from build123d import *

# Parameters (mm, degrees)
F0_R     = 1.875
F1_DEPTH = 11
F2_W     = 17.4188611699
F2_H     = 4.25
F3_DEPTH = 5


# Not quite as in the source:
# - a feature names something its author has since deleted; it is built from what else it names


with BuildPart() as f1:
    # F0 (on Top) → F1 (new body)
    with BuildSketch(Plane.XY):
        with BuildLine():
            ThreePointArc((1.5092688833, -2.1477272727), (2.3294265194, -1.2101227585), (2.625, 0))
            ThreePointArc((2.625, 0), (2.347022952, 1.1756310061), (1.5719651333, 2.1022727273))
            ThreePointArc((1.5719651333, 2.1022727273), (-2.6247144161, 0.0387199415), (1.5092688833, -2.1477272727))
        make_face()
        Circle(F0_R, mode=Mode.SUBTRACT)
        with BuildLine():
            ThreePointArc((1.5719651333, 2.1022727273), (2.347022952, 1.1756310061), (2.625, 0))
            ThreePointArc((2.625, 0), (2.3294265194, -1.2101227585), (1.5092688833, -2.1477272727))
            Line((1.5092688833, -2.1477272727), (24.9281300532, -2.1477272727))
            Line((24.9281300532, -2.1477272727), (24.9281300532, 2.1022727273))
            Line((24.9281300532, 2.1022727273), (1.5719651333, 2.1022727273))
        make_face()
    extrude(amount=F1_DEPTH)

    # F2 (on face) → F3 (join)
    with BuildSketch(Plane.XY.offset(11)):
        with Locations((16.2186994682, -0.0227272727)):
            Rectangle(F2_W, F2_H)
    extrude(amount=F3_DEPTH)


solid = f1.part
Can you work these out from the model? Positions are in its coordinate system, mm. A direction names the side the tool comes from. Give positions to 0.01 mm unless a question says otherwise; leave off trailing zeros. Loops run counter-clockwise (first coordinate to the right, second up) from the corner with the lowest first, then second, coordinate; pieces in that order, holes last. Notation, with made-up numbers: M 28.5,29.5 L 57.5,29.5 A21 ccw 57.5,63.5 Z; hole C 24,18.25 d3. An arc over 180 degrees is marked long. One line per item, written item: value. Start each with the question number.
1) If we section it at A-A, the plane y = 0: Write out the boundary of the cut face in (x, z) (3 decimals).
2) I'm going to push flat-ended pins straight in: pin 1 (1 mm diameter, centred on x = 10.5, y = 0, fed in from -Z); pin 2 (5 mm diameter, centred on x = 9.5, z = 10, fed in from -Y); pin 3 (1.5 mm diameter, centred on y = -2, z = 5.5, fed in from -X). Where does each tip first touch, or does it pass through?
3) If we section it at D-D, the plane x = 8.5: Write out the boundary of the cut face in (y, z).
4) If I drill on line 1 (Y direction, x = 14.5, z = 6); line 2 (Z direction, x = 6.25, y = 1.6); line 3 (X direction, y = -0.7, z = 15), over which ranges is the centre line in solid material (lowest first)? Write a range as [from, to].
5) If we section it at C-C, the plane z = 2.25: Write out the boundary of the cut face in (x, y) (3 decimals).
6) Thinking about a two-plate mould opening in X: for faces 4 (the face through (16, 0, 16)), 5 (the face through (-1.873, 0.082, 5.423)), 6 (the face through (-2.622, 0.119, 5.423)), which applies, +X half, -X half, draft (parallel to the pull), parting line (faces both ways), or undercut?
7) If we section it at B-B, the plane x = 0: Write out the boundary of the cut face in (y, z) (3 decimals), and give its area (3 significant figures).
8) On a 3-axis mill with a long thin cutter (end or side, diameter ignored), from which of +Z, -Z, +X, -X, +Y, -Y can I reach the whole of each face in a straight line? I mean faces 1 (the face through (13, 2.102, 8)), 2 (the face through (13, -2.148, 8)), 3 (the face through (3, 0, 11)). Say none if no direction works.
Completed:
1. outline: M -2.625,0 L -1.875,0 L -1.875,11 L -2.625,11 Z; M 1.875,0 L 24.928,0 L 24.928,16 L 7.509,16 L 7.509,11 L 1.875,11 Z
2. pin 1: stops at z = 0
2. pin 2: stops at y = -2.15
2. pin 3: stops at x = -2.31
3. outline: M -2.15,0 L 2.1,0 L 2.1,16 L -2.15,16 Z
4. line 1: y = [-2.15, 2.1]
4. line 2: z = [0, 11]
4. line 3: x = [7.51, 24.93]
5. outline: M 1.509,-2.148 L 24.928,-2.148 L 24.928,2.102 L 1.572,2.102 A2.625 ccw long Z; hole C 0,0 d3.75
6. face 4: draft
6. face 5: undercut
6. face 6: parting line
7. outline: M -2.625,0 L -1.875,0 L -1.875,11 L -2.625,11 Z; M 1.875,0 L 2.625,0 L 2.625,11 L 1.875,11 Z
7. area: 16.5 mm^2
8. face 1: +Z, -Z, +X, +Y
8. face 2: +Z, -Z, +X, -Y
8. face 3: +Z, -X, +Y, -Y
